Check sheet for the modelled part. Datum: model origin and axes. Units: mm. Face numbers are marked on the shaded views. A direction names the side the tool comes from. Round coordinates to 2 decimals unless told otherwise and drop trailing zeros. Order: outer loops, then holes, each group sorted by start corner. A loop starts at its lowest first (then second) coordinate and runs counter-clockwise, first axis right, second up.
Autodesk Inventor part; units mm, degrees
ref_plane "YZ Plane" through (0, 0, 0) normal (1, 0, 0) x (0, 1, 0)
ref_plane "XZ Plane" through (0, 0, 0) normal (0, 1, 0) x (-1, 0, 0)
ref_plane "XY Plane" through (0, 0, 0) normal (0, 0, 1) x (1, 0, 0)
sketch "草圖1" plane through (0, 0, 0) normal (0, 0, 1) x (1, 0, 0)
  line L0 (0, 0) -> (0, 38)
  line L1 (0, 38) -> (66, 38)
  line L2 (66, 38) -> (120, 8)
  line L3 (120, 8) -> (120, -16)
  line L4 (120, -16) -> (78, -16)
  line L5 (78, -16) -> (78, 0)
  line L6 (78, 0) -> (0, 0)
  dimension "d0" = 54
  dimension "d1" = 38
  dimension "d2" = 24
  dimension "d3" = 42
  dimension "d4" = 66
  dimension "d5" = 120
extrude "擠出1" add sketch "草圖1" against normal blind 54
sketch "草圖2" plane through (0, 38, 0) normal (0, 1, 0) x (1, 0, 0)
  arc A0 (18, 36) -> (18, 20) centre (18, 28) ccw
  line L0 (18, 36) -> (44, 36)
  line L1 (18, 20) -> (44, 20)
  arc A1 (44, 20) -> (44, 36) centre (44, 28) ccw
  line L2 (0, 0) -> (66, 0)
  line L3 (0, 0) -> (0, 54)
  dimension "d8" = 28
  dimension "d9" = 16
  dimension "d10" = 18
  dimension "d11" = 26
extrude "擠出2" cut sketch "草圖2" against normal up to next
sketch "草圖3" plane through (78, -16, 0) normal (0, -1, 0) x (1, 0, 0)
  line L0 (12, -54) -> (12, -40)
  line L1 (12, -40) -> (42, -40)
  line L2 (42, -40) -> (42, -54)
  line L3 (42, -54) -> (12, -54)
  line L4 (42, 0) -> (42, -54)
  line L5 (42, -27) -> (-15.5842, -27)
  line L6 (12, 0) -> (12, -14)
  line L7 (12, -14) -> (42, -14)
  line L8 (42, -14) -> (42, 0)
  line L9 (42, 0) -> (12, 0)
  line L10 (42, -54) -> (42, 0)
  point P0 (-78, 0)
  point P1 (0, 0)
  point P2 (0, -54)
  point P3 (0, 0)
  dimension "d18" = 30
  dimension "d19" = 14
extrude "擠出3" cut sketch "草圖3" against normal up to next
properties part number "410571040-T1"
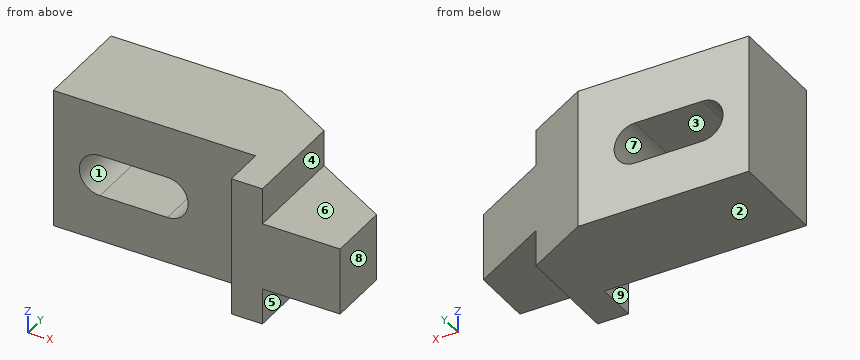
Item 1: Release check for a two-part mould opening along X. For the marked faces 1, 2, 3 and 4 record: released by +X, released by -X, zero draft, split by the parting line, or undercut.
Answer:
face 1: undercut
face 2: zero draft
face 3: undercut
face 4: released by +X
Item 2: Access from +Z, -Z, +X, -X, +Y, -Y to the whole of each face (thin tool, end or side, straight path). Record for the marked faces 5, 6, 7, 8 and 9.
Answer:
face 5: -Z, +X, +Y, -Y
face 6: +Z, +X, +Y, -Y
face 7: +Y, -Y
face 8: +Z, -Z, +X, +Y, -Y
face 9: +Z, -Z, -X, -Y
Item 3: Scan lines: line 1 along Z through (x, y) = (25.5, 2.5); line 2 along Y through (x, z) = (5.5, -4.5); line 3 along X through (y, z) = (13, -29). Record each from-to range of solid material in increasing order.
Answer:
line 1: z = -54 to -36, -20 to 0
line 2: y = 0 to 38
line 3: x = 0 to 10.06, 51.94 to 111
Item 4: Sectioned sample at B-B (y = 13.5). Record the cut outline in (x, z), and give its area (3 significant figures).
Answer:
outline: (0, -54) - (90, -54) - (90, -40) - (110.1, -40) - (110.1, -14) - (90, -14) - (90, 0) - (0, 0) - close; hole (18, -36) - (44, -36) arc R8 ccw to (44, -20) - (18, -20) arc R8 ccw to start
area: 4,770 mm2
Item 5: Sectioned sample at A-A (z = -28). Record the cut outline in (x, y), and give its area (3 significant figures).
Answer:
outline: (0, 0) - (10, 0) - (10, 38) - (0, 38) - close; (52, 0) - (78, 0) - (78, -16) - (120, -16) - (120, 8) - (66, 38) - (52, 38) - close
area: 2,830 mm2
Item 6: Sectioned sample at C-C (y = -9). Record the cut outline in (x, z).
Answer:
outline: (78, -54) - (90, -54) - (90, -40) - (120, -40) - (120, -14) - (90, -14) - (90, 0) - (78, 0) - close
Item 7: Go/stop test with flat-tipped pins: P1, Ø16, axis at x = 37.5, z = -29.5, coming from the -Y side; P2, Ø3, axis at x = 56.5, y = 8, coming from the +Z side; P3, Ø4, axis at y = 6.5, z = -43.5, coming from the +X side; P4, Ø8, axis at y = -4.5, z = -35, coming from the -X side. Record where each tip stops, or that it passes through.
Answer:
P1: stops at y = 0
P2: stops at z = 0
P3: stops at x = 90
P4: stops at x = 78
Item 8: Sectioned sample at D-D (z = -9.5). Record the cut outline in (x, y).
Answer:
outline: (0, 0) - (78, 0) - (78, -16) - (90, -16) - (90, 24.67) - (66, 38) - (0, 38) - close
